Build history of the part. All positions in model axes, mm. A direction names the side the tool comes from. Coordinates: 2 decimals unless noted, no trailing zeros. Order: outer loops, then holes, each group sorted by start corner. A loop starts at its lowest first (then second) coordinate and runs counter-clockwise, first axis right, second up. Notation, with made-up numbers: M 21,10.5 L 79,10.5 A25 cw 79,49.5 Z; hole C 16,49 d7. An arc over 180 degrees is marked long. Write item = value, one per line. Start each with the question number.
Q1. Band-saw the part on C-C on z = 1730. Write the cut outline in (x, y).
Q2. Pull direction Y, two halves, no side cores. Call faces 1 (the face through (-255, -228, 22)), 2 (the face through (-278, 205, 22)), 3 (the face through (-4, 250, 912)), 4 (the face through (277, -205, 22)): released by +Y, released by -Y, zero draft, split by the parting line, or undercut.
Q3. Band-saw the part on B-B on x = -117. Write the cut outline in (y, z).
Q4. 3-axis set-ups, long thin cutter, end or side, ignore diameter. For faces 5 (the face through (277, 205, 22)), 6 (the face through (-4, -225, 969)), 7 (the face through (265, -250, 921)), 8 (the face through (255, -228, 22)): which of +Z, -Z, +X, -X, +Y, -Y reach the whole face in a straight line?
Q5. Band-saw the part on A-A on y = 70.5. Write the cut outline in (x, z).
Q6. Pin check, flat tips, straight feed: P1, Ø10, axis at x = 120, z = 776.5, coming from the -Y side; P2, Ø13.5, axis at x = -270, z = 28, coming from the +Y side; P3, Ø10, axis at y = 210.5, z = 1454.5, coming from the -X side. Stop position of each tip, or through.
Q7. Drill centre lines: probe 1 along Z at (x, y) = (-225, -241); probe 2 along X at (y, z) = (-239.5, 1193.5); probe 3 along X at (y, z) = (98, 601). Where is each one in solid material? Low to high.
```python
from build123d import *

# Parameters (mm, degrees)
F0_W     = 600
F0_H     = 500
F1_DEPTH = 1850
F2_W     = 700
F2_H     = 550
F3_DEPTH = 30
F4_W     = 510
F4_H     = 45
F5_DEPTH = 500
F6_W     = 410
F6_H     = 45
F7_DEPTH = 650.001
F8_W     = 520
F8_H     = 1705
F9_DEPTH = 25


with BuildPart() as f1:
    # F0 (on Top) → F1 (new body)
    with BuildSketch(Plane.XY):
        Rectangle(F0_W, F0_H)
    extrude(amount=F1_DEPTH)

    # F2 (on face) → F3 (join)
    with BuildSketch(Plane.XY.offset(1850)):
        Rectangle(F2_W, F2_H)
    extrude(amount=F3_DEPTH)

    # F4 (on face) → F5 (cut, through all)
    with BuildSketch(Plane.XZ.offset(250)):
        with Locations((0, 22.5)):
            Rectangle(F4_W, F4_H)
    extrude(amount=-F5_DEPTH, mode=Mode.SUBTRACT)

    # F6 (on face) → F7 (cut, through all)
    with BuildSketch(Plane(origin=(-300, 0, 0), x_dir=(0, -1, 0), z_dir=(-1, 0, 0))):
        with Locations((0, 22.5)):
            Rectangle(F6_W, F6_H)
    extrude(amount=-F7_DEPTH, mode=Mode.SUBTRACT)

    # F8 (on face) → F9 (cut)
    with BuildSketch(Plane.XZ.offset(250)):
        with Locations((0, 957.5)):
            Rectangle(F8_W, F8_H)
    extrude(amount=-F9_DEPTH, mode=Mode.SUBTRACT)


solid = f1.part
```
Recorded:
q1.outline = M -300,-250 L -260,-250 L -260,-225 L 260,-225 L 260,-250 L 300,-250 L 300,250 L -300,250 Z
q2.face_1 = zero draft
q2.face_2 = undercut
q2.face_3 = released by +Y
q2.face_4 = undercut
q3.outline = M -275,1850 L -250,1850 L -250,1810 L -225,1810 L -225,105 L -250,105 L -250,45 L 250,45 L 250,1850 L 275,1850 L 275,1880 L -275,1880 Z
q4.face_5 = -Z, +X, -X
q4.face_6 = -Y
q4.face_7 = -Z, +X, -X, -Y
q4.face_8 = -Z, +Y, -Y
q5.outline = M -350,1850 L -300,1850 L -300,45 L 300,45 L 300,1850 L 350,1850 L 350,1880 L -350,1880 Z
q6.P1 = -225
q6.P2 = 250
q6.P3 = -300
q7.probe_1 = 45 to 105, 1810 to 1880
q7.probe_2 = -300 to -260, 260 to 300
q7.probe_3 = -300 to 300
